Part model, mm, in its own coordinate system. A direction names the side the tool comes from. Give positions to 0.01 mm unless a question says otherwise; leave off trailing zeros. Order: outer loops, then holes, each group sorted by start corner. A loop starts at its lowest first (then second) coordinate and runs counter-clockwise, first axis right, second up. Notation, with made-up numbers: M -21.75,50.5 L -11.75,50.5 A29 cw -11.75,89.5 Z; hole C 39,-21.5 d11. An arc over 180 degrees is marked long. Answer as a JSON object with one key per item and string values.
from build123d import *

# Parameters (mm, degrees)
SKETCH_1_W          = 22.5
SKETCH_1_H          = 12
SKETCH_1_W_2        = 20.5
SKETCH_1_H_2        = 10
EXTRUDE_1_DEPTH     = 10
SKETCH_2_W          = 2.5
SKETCH_2_H          = 10
CUT_EXTRUDE_1_DEPTH = 5


with BuildPart() as part:
    # 草图1 → 凸台-拉伸1 (new body)
    with BuildSketch(Plane(origin=(0, 0, 0), x_dir=(1, 0, 0), z_dir=(0, 1, 0))):
        Rectangle(SKETCH_1_W, SKETCH_1_H)
        Rectangle(SKETCH_1_W_2, SKETCH_1_H_2, mode=Mode.SUBTRACT)
    extrude(amount=EXTRUDE_1_DEPTH)

    # 草图2 → 切除-拉伸1 (cut)
    with BuildSketch(Plane(origin=(11.25, 0, 0), x_dir=(0, 0, -1), z_dir=(1, 0, 0))):
        with Locations((0, 5)):
            Rectangle(SKETCH_2_W, SKETCH_2_H)
    extrude(amount=-CUT_EXTRUDE_1_DEPTH, mode=Mode.SUBTRACT)


solid = part.part
1. Cut at C-C on y = 8.5. Give the cut face in (x, z), plus the area to 3 significant figures.
Worked answers:
{"outline": "M -11.25,-6 L 11.25,-6 L 11.25,-1.25 L 10.25,-1.25 L 10.25,-5 L -10.25,-5 L -10.25,5 L 10.25,5 L 10.25,1.25 L 11.25,1.25 L 11.25,6 L -11.25,6 Z", "area": "62.5 mm^2"}
2. Cut at D-D on z = -0.75. Give the cut face in (x, y), plus the area to 3 significant figures.
Worked answers:
{"outline": "M -11.25,0 L -10.25,0 L -10.25,10 L -11.25,10 Z", "area": "10.0 mm^2"}
3. Probe line 1 along Z through (x, y) = (3, 4.5); line 2 along X through (y, z) = (2.25, -2.5); line 3 along X through (y, z) = (8.5, -0.25). List the from-to ranges inside material, lowest first.
Worked answers:
{"line 1": "z = -6 to -5, 5 to 6", "line 2": "x = -11.25 to -10.25, 10.25 to 11.25", "line 3": "x = -11.25 to -10.25"}
4. Cut at B-B on z = 3.75. Give the cut face in (x, y).
Worked answers:
{"outline": "M -11.25,0 L -10.25,0 L -10.25,10 L -11.25,10 Z; M 10.25,0 L 11.25,0 L 11.25,10 L 10.25,10 Z"}
5. Which spindle directions (+Z, -Z, +X, -X, +Y, -Y) get a long thin tool onto all of the face, cutting with end or side? Do faces 1 (the flat face through (0, 5, -5)), 2 (the flat face through (11, 5, 1.25)), 3 (the flat face through (-0.9, 0, -5.4)). Say none if no direction does.
Worked answers:
{"face 1": "+Y, -Y", "face 2": "+X, +Y, -Y", "face 3": "+Z, -Z, +X, -X, -Y"}
6. Pin check, flat tip, straight feed: P1, Ø5, axis at y = 3.5, z = 0, coming from the +X side. Stop position of the tip, or through.
Worked answers:
{"P1": "stops at x = 11.25"}
7. Cut at A-A on x = -6.5. Give the cut face in (y, z).
Worked answers:
{"outline": "M 0,-6 L 10,-6 L 10,-5 L 0,-5 Z; M 0,5 L 10,5 L 10,6 L 0,6 Z"}
8. Two-plate mould, pull along X, no slides. Class faces 4 (the flat face through (0, 5, 5)), 5 (the flat face through (0, 5, 6)), 6 (the flat face through (11.25, 5, -4)): +X half, -X half, draft (parallel to the pull), parting line (faces both ways), or undercut.
Worked answers:
{"face 4": "undercut", "face 5": "draft", "face 6": "+X half"}
